Autodesk Fusion 360 part; units mm, degrees
sketch "Main Body" plane through (0, 0, 0) normal (0, 0, 1) x (1, 0, 0)
  line L0 (123.9438, 6.7249) -> (123.9438, 13.8361)
  arc A0 (117.5938, 0.3749) -> (123.9438, 6.7249) centre (117.5938, 6.7249) ccw
  line L1 (123.9438, 6.7249) -> (64.5078, 6.7249) construction
  line L2 (117.5938, 0.3749) -> (67.3042, 0.3749)
  line L3 (61.0843, 7.1711) -> (27.4293, 7.1711)
  arc A1 (65.0438, 3.571) -> (61.0843, 7.1711) centre (61.0843, 3.1937) ccw
  arc A2 (65.0438, 3.571) -> (67.3042, 0.3749) centre (68.2411, 3.4349) ccw
  circle A3 centre (17.8824, 11.2984) radius 3.175
  line L4 (117.5938, 20.1861) -> (19.8575, 20.1861)
  arc A4 (19.8575, 20.1861) -> (25.3469, 6.0854) centre (17.8824, 11.2984) ccw
  arc A5 (27.4293, 7.1711) -> (25.3469, 6.0854) centre (27.4293, 4.6311) ccw
  arc A6 (123.9438, 13.8361) -> (117.5938, 20.1861) centre (117.5938, 13.8361) ccw
  point P0 (123.9438, 8.0934)
  dimension "d173" = 6.35
  dimension "d175" = 59.436
  dimension "d178" = 6.35
  dimension "d221" = 2.54
  dimension "d223" = 50.2896
  dimension "d229" = 6.35
  dimension "d230" = 33.655
extrude "Extrude2" add sketch "Main Body" along normal blind 10.795
ref_plane "WorkPlane2" through (65.2693, 10.7273, 0) normal (0, 0, -1) x (-1, 0, 0)
sketch "Cut out for Actuator" plane through (0, 0, 0) normal (0, 0, -1) x (-1, 0, 0)
  line L0 (-3.356, 0.6564) -> (-28.756, 0.6564)
  line L1 (-28.756, 0.6564) -> (-28.756, 21.8424)
  line L2 (-28.756, 21.8424) -> (-3.356, 21.8424)
  line L3 (-3.356, 21.8424) -> (-3.356, 0.6564)
  dimension "d205" = 25.4
extrude "Extrude7" cut sketch "Cut out for Actuator" against normal blind 2.54
hole "Hole3" at (109.7706, 10.0261, 0) direction (0, 0, 1) diameter 3.429 depth 8.255 tip angle 180
hole "Hole4" at (81.1448, 10.0261, 0) direction (0, 0, 1) diameter 3.429 depth 8.255 tip angle 180
fillet "Fillet1" radius 1.27 1 faces at (100.8306, 6.9786, 10.795)
The listing builds one solid part. Answer for the finished solid, in the listing's coordinates (mm). A direction names the side the tool comes from. Give positions to 0.01 mm unless a question says otherwise; leave off trailing zeros. Order: outer loops, then holes, each group sorted by start corner. A loop starts at its lowest first (then second) coordinate and runs counter-clockwise, first axis right, second up. Notation, with made-up numbers: (19.25, -16.5) - (77.25, -16.5) arc R19 ccw to (77.25, 2.5) - close; hole circle Ø4 at (65, 7.5). An arc over 180 degrees is marked (long way). One line per item, written item: value. Start each with the question number.
1) Find the intervals of material crossed by L1, parallel to X at y = 11, z = 4; L2, parallel to X at y = 10.5, z = 1.25; L3, parallel to X at y = 7.5, z = 2.25, in increasing order.
2) Given pin 1 Ø3 at (x, z) = (93, 6) entering from +Y; pin 2 Ø2.5 at (x, y) = (109.77, 10.03) entering from -Z (3 decimals); pin 3 Ø1.5 at (y, z) = (14, 2) entering from -X; pin 4 Ø5.5 at (x, y) = (17.88, 11.3) entering from -Z, each flat-ended and moving along its own axis, determine where each tip first touches the part or whether it passes through.
3) A cutting plane is placed at A-A on z = 3.75. State how many separate pieces and enclosed holes the cut face has, then the cut area to 3 significant figures.
4) A cutting plane is placed at B-B on x = 33. Give the vertices of the cut face in (y, z) (3 decimals).
5) The mould has two halves that part along X. Classify faces 5 (the face through (28.756, 14, 1)), 6 (the face through (21, 13, 2.54)), 7 (the face through (9.5, 7.74, 5.98)): released by +X, released by -X, zero draft, split by the parting line, or undercut.
6) A tool of negligible diameter and unlimited length cuts with its end or side. For faces 1 (the face through (63.73, 6.164, 4.696)), 2 (the face through (110, 10, 8.255)), 3 (the face through (69, 20.186, 5)), 4 (the face through (15.5, 9.2, 6)), from which of +Z, -Z, +X, -X, +Y, -Y can it reach the whole face along a straight path? Write none if from no direction.
Answer sheet:
1. L1: x = 8.78 to 14.72, 21.04 to 79.73, 82.56 to 108.36, 111.18 to 123.94
1. L2: x = 28.76 to 79.5, 82.79 to 108.12, 111.42 to 123.94
1. L3: x = 28.76 to 123.94
2. pin 1: stops at y = 20.19
2. pin 2: stops at z = 8.255
2. pin 3: stops at x = 9.04
2. pin 4: passes through
3. separate pieces: 1
3. enclosed holes: 3
3. area: 1,870 mm2
4. outline: (7.171, 0) - (20.186, 0) - (20.186, 9.525) arc R1.27 ccw to (18.916, 10.795) - (8.441, 10.795) arc R1.27 ccw to (7.171, 9.525) - close
5. face 5: released by -X
5. face 6: zero draft
5. face 7: undercut
6. face 1: +Z, -Z, -Y
6. face 2: -Z
6. face 3: +Z, -Z, +X, +Y
6. face 4: +Z, -Z
